Here's how the part is built. I have some questions about the finished solid (model axes, mm). Coordinates: 2 decimals unless noted, no trailing zeros. Loops run counter-clockwise (first coordinate to the right, second up) from the corner with the lowest first, then second, coordinate; pieces in that order, holes last. Notation, with made-up numbers: (8, 51.5) -> (47, 51.5) arc R28 ccw to (47, 72.5) -> close; hole circle Ø6 at (-25.75, 76.25). An arc over 180 degrees is marked (long way). Answer as a JSON object with one key per item and string values. Group by question number.
Q1. I want a section at B-B on y = -47.5. Write out the boundary of the cut face in (x, z) (3 decimals).
Q2. I want a section at D-D on z = 0.7. Count the separate pieces of the cut face and the enclosed holes in it, then the cut area to 3 significant figures.
Q3. I need wall thicknesses on line 1 (X direction, y = -46.5, z = 0.3) (3 decimals); line 2 (Y direction, x = 26, z = 0.5) (3 decimals); line 3 (Y direction, x = 43, z = 1.4) (3 decimals). Which ranges of each line are inside material? Lowest first, please.
Q4. I want a section at C-C on y = -0.5. Write out the boundary of the cut face in (x, z).
Q5. I want a section at A-A on x = 67. Write out the boundary of the cut face in (y, z) (3 decimals), then the cut area to 3 significant figures.
Autodesk Fusion 360 part; units mm, degrees
sketch "plate-2026-01-04T06_23_53.757Z" plane through (0, 0, 0) normal (0, 0, 1) x (1, 0, 0)
  line L0 (3.025, -40.625) -> (16.025, -40.625)
  line L1 (3.025, -54.625) -> (16.025, -54.625)
  line L2 (2.525, -41.125) -> (2.525, -54.125)
  line L3 (16.525, -41.125) -> (16.525, -54.125)
  arc A0 (3.025, -40.625) -> (2.525, -41.125) centre (3.025, -41.125) ccw
  arc A1 (16.525, -41.125) -> (16.025, -40.625) centre (16.025, -41.125) ccw
  arc A2 (2.525, -54.125) -> (3.025, -54.625) centre (3.025, -54.125) ccw
  arc A3 (16.025, -54.625) -> (16.525, -54.125) centre (16.025, -54.125) ccw
  line L4 (22.075, -40.625) -> (35.075, -40.625)
  line L5 (22.075, -54.625) -> (35.075, -54.625)
  line L6 (21.575, -41.125) -> (21.575, -54.125)
  line L7 (35.575, -41.125) -> (35.575, -54.125)
  arc A4 (22.075, -40.625) -> (21.575, -41.125) centre (22.075, -41.125) ccw
  arc A5 (35.575, -41.125) -> (35.075, -40.625) centre (35.075, -41.125) ccw
  arc A6 (21.575, -54.125) -> (22.075, -54.625) centre (22.075, -54.125) ccw
  arc A7 (35.075, -54.625) -> (35.575, -54.125) centre (35.075, -54.125) ccw
  line L8 (41.125, -40.625) -> (54.125, -40.625)
  line L9 (41.125, -54.625) -> (54.125, -54.625)
  line L10 (40.625, -41.125) -> (40.625, -54.125)
  line L11 (54.625, -41.125) -> (54.625, -54.125)
  arc A8 (41.125, -40.625) -> (40.625, -41.125) centre (41.125, -41.125) ccw
  arc A9 (54.625, -41.125) -> (54.125, -40.625) centre (54.125, -41.125) ccw
  arc A10 (40.625, -54.125) -> (41.125, -54.625) centre (41.125, -54.125) ccw
  arc A11 (54.125, -54.625) -> (54.625, -54.125) centre (54.125, -54.125) ccw
  line L12 (60.175, -40.625) -> (73.175, -40.625)
  line L13 (60.175, -54.625) -> (73.175, -54.625)
  line L14 (59.675, -41.125) -> (59.675, -54.125)
  line L15 (73.675, -41.125) -> (73.675, -54.125)
  arc A12 (60.175, -40.625) -> (59.675, -41.125) centre (60.175, -41.125) ccw
  arc A13 (73.675, -41.125) -> (73.175, -40.625) centre (73.175, -41.125) ccw
  arc A14 (59.675, -54.125) -> (60.175, -54.625) centre (60.175, -54.125) ccw
  arc A15 (73.175, -54.625) -> (73.675, -54.125) centre (73.175, -54.125) ccw
  line L16 (-10.823, 8.872) -> (87.977, 8.872)
  line L17 (87.977, 8.872) -> (87.977, -67.928)
  line L18 (87.977, -67.928) -> (-10.823, -67.928)
  line L19 (-10.823, -67.928) -> (-10.823, 8.872)
  circle A16 centre (-5.823, 3.872) radius 1.7
  circle A17 centre (82.977, 3.872) radius 1.7
  circle A18 centre (82.977, -62.928) radius 1.7
  circle A19 centre (-5.823, -62.928) radius 1.7
  line L20 (30.232, 8.872) -> (48.732, 8.872)
  line L21 (48.732, 8.872) -> (48.732, -22.128)
  line L22 (48.732, -22.128) -> (30.232, -22.128)
  line L23 (30.232, -22.128) -> (30.232, 8.872)
  circle A20 centre (9.427, -8.428) radius 4
  circle A21 centre (68.227, -8.428) radius 4
  line L24 (18.992, -24.543) -> (56.992, -24.543)
  line L25 (56.992, -24.543) -> (56.992, -36.543)
  line L26 (56.992, -36.543) -> (18.992, -36.543)
  line L27 (18.992, -36.543) -> (18.992, -24.543)
  dimension "d1" = 76.8
  dimension "d2" = 98.8
  dimension "d3" = 13.348
  dimension "d4" = 13.303
  dimension "d5" = 3.4
  dimension "d6" = 5
  dimension "d7" = 5
  dimension "d8" = 3.4
  dimension "d9" = 5
  dimension "d10" = 5
  dimension "d11" = 3.4
  dimension "d12" = 5
  dimension "d13" = 5
  dimension "d14" = 3.4
  dimension "d15" = 5
  dimension "d16" = 5
  dimension "d17" = 31
  dimension "d18" = 18.5
  dimension "d19" = 41.055
  dimension "d20" = 8
  dimension "d21" = 17.3
  dimension "d22" = 20.25
  dimension "d23" = 8
  dimension "d24" = 17.3
  dimension "d25" = 19.75
  dimension "d26" = 12
  dimension "d27" = 38
  dimension "d28" = 29.815
  dimension "d29" = 31.385
extrude "Extrude1" add sketch "plate-2026-01-04T06_23_53.757Z" along normal blind 1.5 contours L16 L17 L18 L19 L21 L22 L23
fillet "Fillet1" radius 5 1 edges at (87.977, 8.872, 0.75)
fillet "Fillet2" radius 5 1 edges at (-10.823, 8.872, 0.75)
fillet "Fillet3" radius 5 1 edges at (-10.823, -67.928, 0.75)
fillet "Fillet4" radius 5 1 edges at (87.977, -67.928, 0.75)
equation "d3 = 9.5 mm + 3.848 mm"
equation "d4 = 3.803 mm + 9.5 mm"
equation "d19 = 35.305 mm + 5.75 mm"
equation "d21 = 7.8 mm + 9.5 mm"
equation "d22 = 9.5 mm + 10.75 mm"
equation "d24 = 9.5 mm + 7.8 mm"
equation "d25 = 9.5 mm + 10.250 mm"
equation "d28 = 9.5 mm + 20.315 mm"
equation "d29 = 21.885 mm + 9.5 mm"
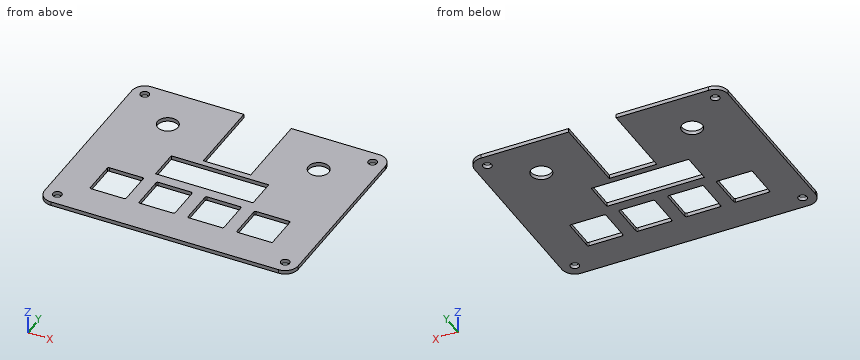
Result set:
{
 "1": {"outline": "(-10.823, 0) -> (2.525, 0) -> (2.525, 1.5) -> (-10.823, 1.5) -> close; (16.525, 0) -> (21.575, 0) -> (21.575, 1.5) -> (16.525, 1.5) -> close; (35.575, 0) -> (40.625, 0) -> (40.625, 1.5) -> (35.575, 1.5) -> close; (54.625, 0) -> (59.675, 0) -> (59.675, 1.5) -> (54.625, 1.5) -> close; (73.675, 0) -> (87.977, 0) -> (87.977, 1.5) -> (73.675, 1.5) -> close"},
 "2": {"separate pieces": "1", "enclosed holes": "11", "area": "5,620 mm²"},
 "3": {"line 1": "x = -10.823 to 2.525, 16.525 to 21.575, 35.575 to 40.625, 54.625 to 59.675, 73.675 to 87.977", "line 2": "y = -67.928 to -54.625, -40.625 to -36.543, -24.543 to 8.872", "line 3": "y = -67.928 to -54.625, -40.625 to -36.543, -24.543 to -22.128"},
 "4": {"outline": "(-10.82, 0) -> (30.23, 0) -> (30.23, 1.5) -> (-10.82, 1.5) -> close; (48.73, 0) -> (87.98, 0) -> (87.98, 1.5) -> (48.73, 1.5) -> close"},
 "5": {"outline": "(-67.928, 0) -> (-54.625, 0) -> (-54.625, 1.5) -> (-67.928, 1.5) -> close; (-40.625, 0) -> (-12.235, 0) -> (-12.235, 1.5) -> (-40.625, 1.5) -> close; (-4.621, 0) -> (8.872, 0) -> (8.872, 1.5) -> (-4.621, 1.5) -> close", "area": "82.8 mm²"}
}
